Here's the drawing with two shaded views (mm, measured from the low corner). I have some questions. Round coordinates to 2 decimals unless told otherwise and drop trailing zeros. Order: outer loops, then holes, each group sorted by start corner. A loop starts at its lowest first (then second) coordinate and runs counter-clockwise, first axis right, second up.
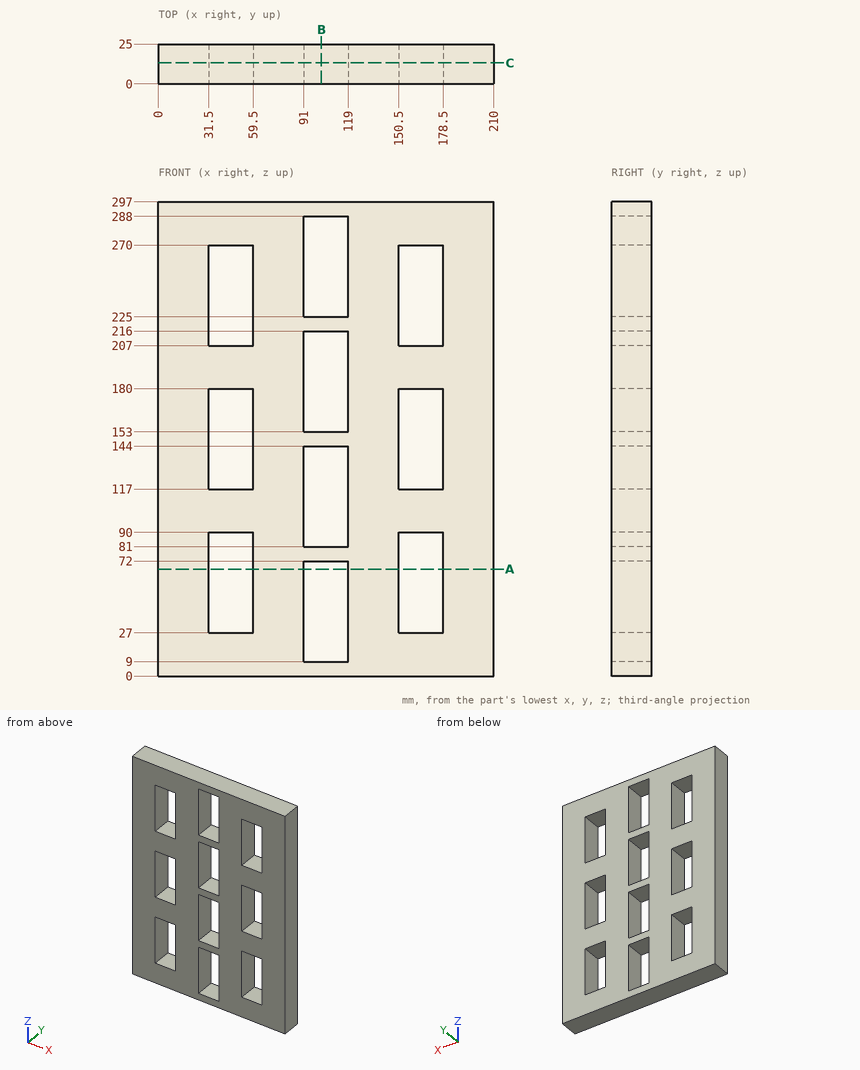
1. If we section it at A-A, the plane z = 67: Write out the boundary of the cut face in (x, y), and give its area (3 significant figures).
Evaluation:
outline: (0, 0) - (31.5, 0) - (31.5, 25) - (0, 25) - close; (59.5, 0) - (91, 0) - (91, 25) - (59.5, 25) - close; (119, 0) - (150.5, 0) - (150.5, 25) - (119, 25) - close; (178.5, 0) - (210, 0) - (210, 25) - (178.5, 25) - close
area: 3,150 mm2
2. If we section it at C-C, the plane y = 13.25: State how many separate pieces and enclosed holes the cut face has, and give its area (3 significant figures).
Evaluation:
separate pieces: 1
enclosed holes: 10
area: 44,700 mm2
3. I need wall thicknesses on probe 1 along X at (y, z) = (15, 30); probe 2 along Z at (x, y) = (176.5, 8); probe 3 along X at (y, z) = (22.25, 151). Which ranges of each line are inside material? Lowest first, please.
Evaluation:
probe 1: x = 0 to 31.5, 59.5 to 91, 119 to 150.5, 178.5 to 210
probe 2: z = 0 to 27, 90 to 117, 180 to 207, 270 to 297
probe 3: x = 0 to 31.5, 59.5 to 150.5, 178.5 to 210
4. I'm going to push a flat-ended pin straight in: P1, Ø12.5, axis at y = 10, z = 237, coming from the -X side. Where does the tip first touch, or does it pass through?
Evaluation:
P1: stops at x = 0
5. If we section it at B-B, the plane x = 102: Write out the boundary of the cut face in (y, z).
Evaluation:
outline: (0, 0) - (25, 0) - (25, 9) - (0, 9) - close; (0, 72) - (25, 72) - (25, 81) - (0, 81) - close; (0, 144) - (25, 144) - (25, 153) - (0, 153) - close; (0, 216) - (25, 216) - (25, 225) - (0, 225) - close; (0, 288) - (25, 288) - (25, 297) - (0, 297) - close
